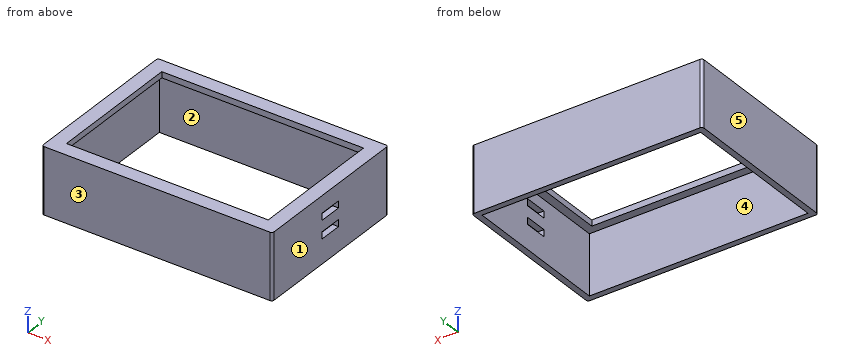
```python
from build123d import *

# Parameters (mm, degrees)
SKETCH1_W           = 96
SKETCH1_H           = 68
SKETCH1_W_2         = 84
SKETCH1_H_2         = 56
BOSS_EXTRUDE1_DEPTH = 2.5
SKETCH2_W           = 96
SKETCH2_H           = 68
SKETCH2_W_2         = 91
SKETCH2_H_2         = 63
BOSS_EXTRUDE2_DEPTH = 25
FILLET1_R           = 1
SKETCH3_W           = 2.865098433
SKETCH3_H           = 9.669707212
CUT_EXTRUDE1_DEPTH  = 2.5


with BuildPart() as part:
    # Sketch1 → Boss-Extrude1 (new body)
    with BuildSketch(Plane.XY):
        Rectangle(SKETCH1_W, SKETCH1_H)
        Rectangle(SKETCH1_W_2, SKETCH1_H_2, mode=Mode.SUBTRACT)
    extrude(amount=-BOSS_EXTRUDE1_DEPTH)

    # Sketch2 → Boss-Extrude2 (add)
    with BuildSketch(Plane(origin=(0, 0, -2.5), x_dir=(-1, 0, 0), z_dir=(0, 0, -1))):
        Rectangle(SKETCH2_W, SKETCH2_H)
        Rectangle(SKETCH2_W_2, SKETCH2_H_2, mode=Mode.SUBTRACT)
    extrude(amount=BOSS_EXTRUDE2_DEPTH)

    # Fillet1
    fillet1_edges = [part.edges().sort_by_distance(p)[0] for p in [
        (-48, 34, -13.75),
        (48, 34, -13.75),
        (48, -34, -13.75),
        (-48, -34, -13.75),
    ]]
    fillet(fillet1_edges, radius=FILLET1_R)

    # Sketch3 → Cut-Extrude1 (cut)
    with BuildSketch(Plane(origin=(48, 0, 0), x_dir=(0, 0, -1), z_dir=(1, 0, 0))):
        with Locations((15.997319539, 0)):
            Rectangle(SKETCH3_W, SKETCH3_H)
        with Locations((8.497319539, 0)):
            Rectangle(SKETCH3_W, SKETCH3_H)
    extrude(amount=-CUT_EXTRUDE1_DEPTH, mode=Mode.SUBTRACT)


solid = part.part
```
Verification items for the finished model (mm, model axes). Face numbers are marked on the shaded views. A direction names the side the tool comes from. Coordinates: 2 decimals unless noted, no trailing zeros. Loops run counter-clockwise (first coordinate to the right, second up) from the corner with the lowest first, then second, coordinate; pieces in that order, holes last. Notation, with made-up numbers: (-25.5, -6.75) -> (28.5, -6.75) arc R19 cw to (28.5, -2.75) -> close; hole circle Ø9 at (17.5, 71.25). An arc over 180 degrees is marked (long way). Answer in a Markdown table with one row per item. Add a question column.
1. Access from +Z, -Z, +X, -X, +Y, -Y to the whole of each face (thin tool, end or side, straight path). Record for the marked faces 1 and 2.
2. Depth check by flat-ended pin: P1, Ø5, axis at x = -3, y = 26, coming from the -Z side. Enter the tip coordinate at first touch or a pass-through.
3. Section check A-A, the plane y = -25. Enter the section's corners in (x, z), then the cut area to 3 significant figures.
4. Section check D-D, the plane z = -16.25. Enter the section's corners in (x, y), then the cut area to 3 significant figures.
5. Section check C-C, the plane z = -5. Enter the section's corners in (x, y).
6. Draft check along Y on the marked faces 3, 4 and 5. Enter one of: +Y half, -Y half, draft (parallel to the pull), parting line (faces both ways), or undercut.
7. Section check B-B, the plane x = -18.5. Enter the section's corners in (y, z).
8. Material ranges on probe 1 along X at (y, z) = (7.5, -8); probe 2 along X at (y, z) = (-12.5, -1.75); probe 3 along Y at (x, z) = (34, -17.75), recorded low to high. Write a range as [from, to].
Derived:
| question | item | result |
|---|---|---|
| 1 | face 1 | +Z, -Z, +X, +Y, -Y |
| 1 | face 2 | -Z |
| 2 | P1 | stops at z = -2.5 |
| 3 | outline | (-48, -27.5) -> (-45.5, -27.5) -> (-45.5, -2.5) -> (-42, -2.5) -> (-42, 0) -> (-48, 0) -> close; (42, -2.5) -> (45.5, -2.5) -> (45.5, -27.5) -> (48, -27.5) -> (48, 0) -> (42, 0) -> close |
| 3 | area | 155 mm² |
| 4 | outline | (-48, -33) arc R1 ccw to (-47, -34) -> (47, -34) arc R1 ccw to (48, -33) -> (48, -4.83) -> (45.5, -4.83) -> (45.5, -31.5) -> (-45.5, -31.5) -> (-45.5, 31.5) -> (45.5, 31.5) -> (45.5, 4.83) -> (48, 4.83) -> (48, 33) arc R1 ccw to (47, 34) -> (-47, 34) arc R1 ccw to (-48, 33) -> close |
| 4 | area | 770 mm² |
| 5 | outline | (-48, -33) arc R1 ccw to (-47, -34) -> (47, -34) arc R1 ccw to (48, -33) -> (48, 33) arc R1 ccw to (47, 34) -> (-47, 34) arc R1 ccw to (-48, 33) -> close; hole (-45.5, -31.5) -> (45.5, -31.5) -> (45.5, 31.5) -> (-45.5, 31.5) -> close |
| 6 | face 3 | -Y half |
| 6 | face 4 | undercut |
| 6 | face 5 | draft |
| 7 | outline | (-34, -27.5) -> (-31.5, -27.5) -> (-31.5, -2.5) -> (-28, -2.5) -> (-28, 0) -> (-34, 0) -> close; (28, -2.5) -> (31.5, -2.5) -> (31.5, -27.5) -> (34, -27.5) -> (34, 0) -> (28, 0) -> close |
| 8 | probe 1 | x = [-48, -45.5], [45.5, 48] |
| 8 | probe 2 | x = [-48, -42], [42, 48] |
| 8 | probe 3 | y = [-34, -31.5], [31.5, 34] |
